Verification items for this drawing (mm, ordinates from the low corner). A direction names the side the tool comes from. Coordinates: 2 decimals unless noted, no trailing zeros. Write each loop counter-clockwise with the first axis right and the second up, starting at its lowest first coordinate (ties: lowest second). Pieces come first, ordered by that corner, then holes. Notation, with made-up numbers: M 56,34.5 L 109,34.5 A16 cw 109,45.5 Z; hole C 3,27 d11. An arc over 180 degrees is marked long. Put each result on its own line as item: value. Start each with the question number.
1) Cross-section at A-A on z = 22. Record the cut outline in (x, y).
2) Mould release check, pull along Z, two halves, no side actions. Record for the marked faces 1, 2 and 3: released by +Z, released by -Z, zero draft, split by the parting line, or undercut.
3) Gauge pin test, flat end, axial feed: pin 1 (6.5 mm diameter, centred on x = 15, z = 12.5, fed in from +Y). Record the tip position at first contact, or that the pin passes through.
4) Cross-section at B-B on x = 35. Record the cut outline in (y, z).
5) Cross-section at D-D on z = 12.5. Count the separate pieces of the cut face and the enclosed holes in it, plus the area to 3 significant figures.
6) Scan lines: line 1 along Y through (x, z) = (42, 8); line 2 along Z through (x, y) = (50.5, 52.5); line 3 along X through (y, z) = (58.9, 12.5). Record each from-to range of solid material in increasing order.
7) Set-up check for the marked faces 4 and 5: record each of +Z, -Z, +X, -X, +Y, -Y from which the full face is reachable in a straight line by a thin tool's end or side.
8) Cross-section at C-C on y = 30. Record the cut outline in (x, z), plus the area to 3 significant figures.
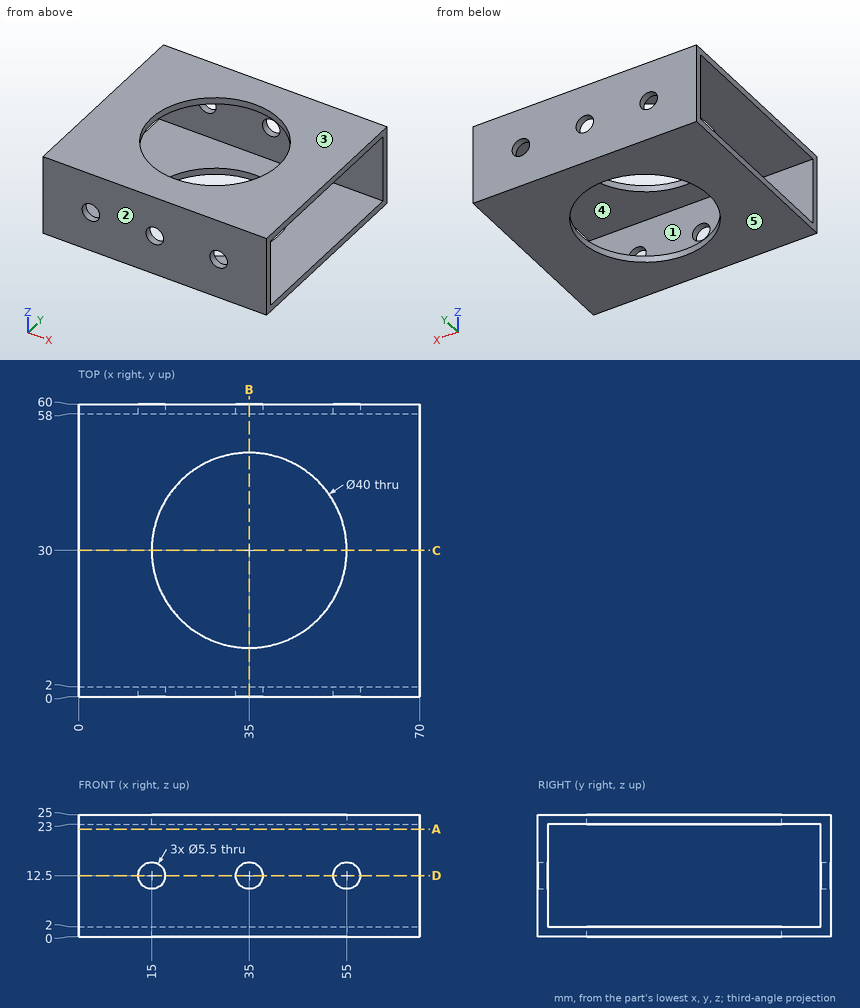
Answer key:
1. outline: M 0,0 L 70,0 L 70,2 L 0,2 Z; M 0,58 L 70,58 L 70,60 L 0,60 Z
2. face 1: undercut
2. face 2: zero draft
2. face 3: released by +Z
3. pin 1: stops at y = 60
4. outline: M 0,0 L 10,0 L 10,2 L 2,2 L 2,9.75 L 0,9.75 Z; M 0,15.25 L 2,15.25 L 2,23 L 10,23 L 10,25 L 0,25 Z; M 50,0 L 60,0 L 60,9.75 L 58,9.75 L 58,2 L 50,2 Z; M 50,23 L 58,23 L 58,15.25 L 60,15.25 L 60,25 L 50,25 Z
5. separate pieces: 8
5. enclosed holes: 0
5. area: 214 mm²
6. line 1: y = 0 to 2, 58 to 60
6. line 2: z = 0 to 2, 23 to 25
6. line 3: x = 0 to 12.25, 17.75 to 32.25, 37.75 to 52.25, 57.75 to 70
7. face 4: +X, -X
7. face 5: -Z, +X, -X, +Y, -Y
8. outline: M 0,0 L 15,0 L 15,2 L 0,2 Z; M 0,23 L 15,23 L 15,25 L 0,25 Z; M 55,0 L 70,0 L 70,2 L 55,2 Z; M 55,23 L 70,23 L 70,25 L 55,25 Z
8. area: 120 mm²
